Here's the drawing with two shaded views (mm, measured from the low corner). I have some questions. A direction names the side the tool comes from. Round coordinates to 2 decimals unless told otherwise and drop trailing zeros. Loops run counter-clockwise (first coordinate to the right, second up) from the corner with the lowest first, then second, coordinate; pieces in that order, holes last. Notation, with made-up numbers: (55, 17) - (107, 17) arc R22 cw to (107, 54) - close; hole circle Ø11 at (29.25, 14.25). An arc over 180 degrees is marked (long way). Answer as CSV lines item,"result".
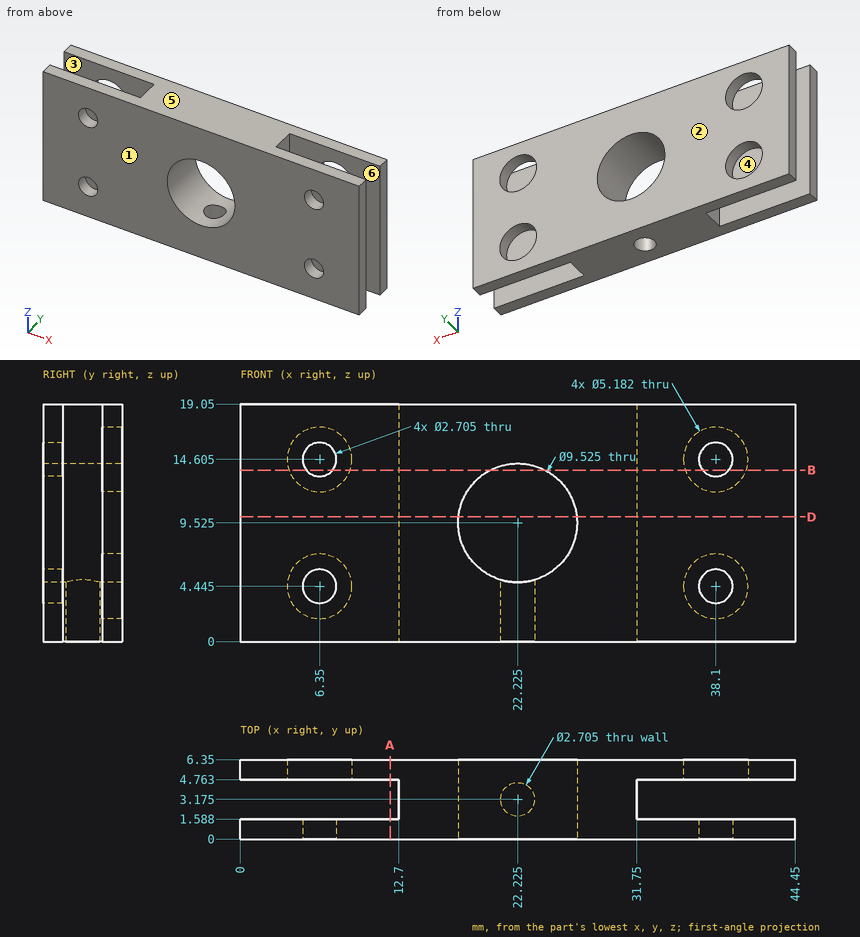
Q1. We'd pull the mould along Y, two halves only. Please class the marked faces 1, 2 and 3: pulls with the +Y half, pulls with the -Y half, needs draft (parallel to the pull), parting line crosses it, or undercut.
Checks:
face 1,"pulls with the -Y half"
face 2,"pulls with the +Y half"
face 3,"undercut"
Q2. Imagine slicing it at D-D (z = 10). Write out the boundary of the cut face in (x, y).
Checks:
outline,"(0, 0) - (17.49, 0) - (17.49, 6.35) - (0, 6.35) - (0, 4.76) - (12.7, 4.76) - (12.7, 1.59) - (0, 1.59) - close; (26.96, 0) - (44.45, 0) - (44.45, 1.59) - (31.75, 1.59) - (31.75, 4.76) - (44.45, 4.76) - (44.45, 6.35) - (26.96, 6.35) - close"
Q3. Imagine slicing it at B-B (z = 13.75). Count the separate pieces of the cut face and the enclosed holes in it.
Checks:
separate pieces,"6"
enclosed holes,"0"
Q4. I'm going to push flat-ended pins straight in: pin 1 Ø8 at (x, z) = (39.5, 6) entering from +Y; pin 2 Ø2.5 at (x, y) = (22.225, 3.175) entering from -Z; pin 3 Ø4.5 at (x, z) = (38.1, 14.605) entering from +Y; pin 4 Ø1.6 at (y, z) = (3, 14) entering from -X. Where does each tip first touch, or does it pass through?
Checks:
pin 1,"y = 6.35"
pin 2,"z = 14.12"
pin 3,"y = 1.59"
pin 4,"x = 12.7"
Q5. If I drill on line 1 along Y through (x, z) = (4, 12); line 2 along Z through (x, y) = (38.1, 0.75); line 3 along X through (y, z) = (0.75, 9.5), over which ranges is the centre line in solid material (lowest first)? Write a range as [from, to].
Checks:
line 1,"[0, 1.59], [4.76, 6.35]"
line 2,"[0, 3.09], [5.8, 13.25], [15.96, 19.05]"
line 3,"[0, 17.46], [26.99, 44.45]"
Q6. On a 3-axis mill with a long thin cutter (end or side, diameter ignored), from which of +Z, -Z, +X, -X, +Y, -Y can I reach the whole of each face in a straight line? I mean the marked faces 4, 5 and 6. Say none if no direction works.
Checks:
face 4,"+Z, -Z, -X"
face 5,"+Z, +X, -X, +Y, -Y"
face 6,"+Z, -Z, +X"
Q7. Imagine slicing it at A-A (x = 12). Write out the boundary of the cut face in (y, z).
Checks:
outline,"(0, 0) - (1.59, 0) - (1.59, 19.05) - (0, 19.05) - close; (4.76, 0) - (6.35, 0) - (6.35, 19.05) - (4.76, 19.05) - close"
